Could you check a few things on this model? Use its own coordinates, in mm. A direction names the side the tool comes from. Coordinates: 2 decimals unless noted, no trailing zeros. Order: outer loops, then holes, each group sorted by start corner. A loop starts at its lowest first (then second) coordinate and runs counter-clockwise, first axis right, second up. Notation, with made-up numbers: (60.25, 44) - (118.25, 44) arc R16 ccw to (118.25, 69) - close; hole circle Ø11 at (-32.75, -15). An arc over 180 degrees is marked (long way). Answer as a JSON object with one key per item and string values. Group by question number.
(1) Which directions (+Z, -Z, +X, -X, +Y, -Y) give clear straight access to the entire face, cutting with the end or side of a thin tool? Please do faces 4 (the flat face through (58, 5.17, 2)), 5 (the flat face through (59.182, 24, 2)), 6 (the flat face through (8, 27.522, 2)), 7 (the flat face through (41.275, 8, 2)), 8 (the flat face through (3.048, 9, 2)).
(2) Please list where these lines run through material, in increasing order: probe 1 along X at (y, z) = (3, 2.9) (3 decimals); probe 2 along X at (y, z) = (8, 1) (3 decimals); probe 3 along X at (y, z) = (22.5, 1.15).
(3) Imagine slicing it at C-C, the plane x = 40. Write out the boundary of the cut face in (y, z), and give its area (3 significant figures).
(4) Imagine slicing it at B-B, the plane y = 12. Write out the boundary of the cut face in (x, z), and give its area (3 significant figures).
(5) Will these pins go through, and if not, where does the flat tip stop? P1, Ø1.5, axis at y = 29.5, z = 2, coming from the +X side (3 decimals); P2, Ø0.9, axis at y = 24, z = 1.5, coming from the -X side; P3, Ø0.9, axis at x = 57, z = 2, coming from the -Y side.
(6) We'd pull the mould along X, two halves only. Please class faces 1 (the flat face through (7.445, 1.267, 1.503)), 2 (the flat face through (17.785, 3, 2)), 3 (the flat face through (12, 0, 2)): pulls with the +X half, pulls with the -X half, needs draft (parallel to the pull), parting line crosses it, or undercut.
from build123d import *

# Parameters (mm, degrees)
BOSS_EXTRUDE1_DEPTH = 3.048


with BuildPart() as part:
    # Model → Boss-Extrude1 (new body)
    with BuildSketch(Plane.XY):
        with BuildLine():
            Line((59.181999415, 5.17), (59.181999415, 13.297999725))
            Line((59.181999415, 13.297999725), (62.229999341, 13.297999725))
            Line((62.229999341, 13.297999725), (62.229999341, 19.597199261))
            Line((62.229999341, 19.597199261), (59.181999415, 19.597199261))
            Line((59.181999415, 19.597199261), (59.181999415, 27.522))
            Line((59.181999415, 27.522), (48.894999549, 27.522))
            Line((48.894999549, 27.522), (48.894999549, 30.696999729))
            Line((48.894999549, 30.696999729), (13.335000724, 30.696999729))
            Line((13.335000724, 30.696999729), (13.335000724, 27.522))
            Line((13.335000724, 27.522), (3.047998995, 27.522))
            Line((3.047998995, 27.522), (3.047998995, 19.597199261))
            Line((3.047998995, 19.597199261), (0, 19.597199261))
            Line((0, 19.597199261), (0, 13.297999725))
            Line((0, 13.297999725), (3.047998995, 13.297999725))
            Line((3.047998995, 13.297999725), (3.047998995, 5.17))
            Line((3.047998995, 5.17), (6.21299938, 5.17))
            Line((6.21299938, 5.17), (6.21299938, 2.5))
            Line((6.21299938, 2.5), (8.71299938, 0))
            Line((8.71299938, 0), (16.28499938, 0))
            ThreePointArc((16.28499938, 0), (17.345659551, 0.439339828), (17.78499938, 1.5))
            Line((17.78499938, 1.5), (17.78499938, 5.17))
            Line((17.78499938, 5.17), (23.799799458, 5.17))
            Line((23.799799458, 5.17), (23.799799458, 10.34))
            Line((23.799799458, 10.34), (41.274999458, 10.34))
            Line((41.274999458, 10.34), (41.274999458, 5.17))
            Line((41.274999458, 5.17), (44.444999458, 5.17))
            Line((44.444999458, 5.17), (44.444999458, 1.5))
            ThreePointArc((44.444999458, 1.5), (44.884339286, 0.439339828), (45.944999458, 0))
            Line((45.944999458, 0), (53.516999458, 0))
            Line((53.516999458, 0), (56.016999458, 2.5))
            Line((56.016999458, 2.5), (56.016999458, 5.17))
            Line((56.016999458, 5.17), (59.181999415, 5.17))
        make_face()
    extrude(amount=BOSS_EXTRUDE1_DEPTH)


solid = part.part
Result set:
{
 "1": {"face 4": "+Z, -Z, +X, -Y", "face 5": "+Z, -Z, +X, +Y", "face 6": "+Z, -Z, -X, +Y", "face 7": "+Z, -Z, -Y", "face 8": "+Z, -Z, -X, -Y"},
 "2": {"probe 1": "x = 6.213 to 17.785, 44.445 to 56.017", "probe 2": "x = 3.048 to 23.8, 41.275 to 59.182", "probe 3": "x = 3.05 to 59.18"},
 "3": {"outline": "(10.34, 0) - (30.7, 0) - (30.7, 3.05) - (10.34, 3.05) - close", "area": "62.0 mm^2"},
 "4": {"outline": "(3.05, 0) - (59.18, 0) - (59.18, 3.05) - (3.05, 3.05) - close", "area": "171 mm^2"},
 "5": {"P1": "stops at x = 48.895", "P2": "stops at x = 3.05", "P3": "stops at y = 5.17"},
 "6": {"face 1": "pulls with the -X half", "face 2": "undercut", "face 3": "needs draft"}
}
